```python
from build123d import *

# Parameters (mm, degrees)
SKETCH_1_R      = 2
EXTRUDE_1_DEPTH = 5.6
FILLET_1_R      = 2
FILLET_2_R      = 2
FILLET_3_R      = 50


with BuildPart() as part:
    # ｽｹｯﾁ1 → ﾎﾞｽ - 押し出し1 (new body)
    with BuildSketch(Plane(origin=(0, 0, 0), x_dir=(1, 0, 0), z_dir=(0, 1, 0))):
        with BuildLine():
            Line((47.5, -35), (67.5, -58.4))
            Line((67.5, -58.4), (67.5, -108.4))
            Line((67.5, -108.4), (36.64, -142.480487319))
            Line((36.64, -142.480487319), (36.64, -172))
            Line((36.64, -172), (-13.36, -172))
            Line((-13.36, -172), (-13.36, -106.551632211))
            ThreePointArc((-13.36, -106.551632211), (45.682817739, -101.546532593), (0, -63.808150114))
            Line((0, -63.808150114), (0, 0))
            Line((0, 0), (37.5, 0))
            Line((37.5, 0), (37.5, -15))
            Line((37.5, -15), (47.5, -15))
            Line((47.5, -15), (47.5, -35))
        make_face()
        with Locations(Location((42.5, -25, 0), (0, 0, 270))):
            Circle(SKETCH_1_R, mode=Mode.SUBTRACT)
        with Locations(Location((42.5, -51, 0), (0, 0, 270))):
            Circle(SKETCH_1_R, mode=Mode.SUBTRACT)
    extrude(amount=EXTRUDE_1_DEPTH)

    # ﾌｨﾚｯﾄ1
    fillet_1_edges = [part.edges().sort_by_distance(p)[0] for p in [
        (-13.36, 2.8, 106.551632211),
        (0, 2.8, 63.808150114),
    ]]
    fillet(fillet_1_edges, radius=FILLET_1_R)

    # ﾌｨﾚｯﾄ2
    fillet_2_edges = [part.edges().sort_by_distance(p)[0] for p in [
        (0, 2.8, 0),
        (37.5, 2.8, 0),
        (47.5, 2.8, 15),
        (67.5, 2.8, 58.4),
        (67.5, 2.8, 108.4),
        (36.64, 2.8, 172),
        (-13.36, 2.8, 172),
    ]]
    fillet(fillet_2_edges, radius=FILLET_2_R)

    # ﾌｨﾚｯﾄ3
    fillet_3_edges = [part.edges().sort_by_distance(p)[0] for p in [
        (36.64, 2.8, 142.480487319),
    ]]
    fillet(fillet_3_edges, radius=FILLET_3_R)


solid = part.part
```
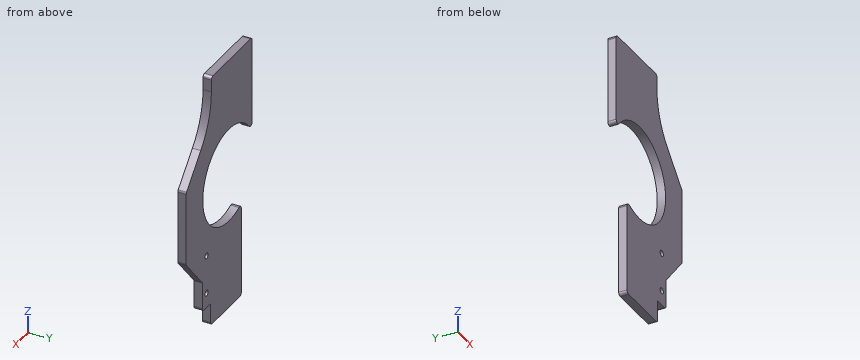
Read the model definition and answer for the solid it produces. Units are mm, in the model's axes. Coordinates: 2 decimals unless noted, no trailing zeros. Loops run counter-clockwise (first coordinate to the right, second up) from the corner with the lowest first, then second, coordinate; pieces in that order, holes last. Notation, with made-up numbers: (-12.75, 38) -> (36.25, 38) arc R35 ccw to (36.25, 75) -> close; hole circle Ø11 at (48, 31.5). An arc over 180 degrees is marked (long way). Return JSON: item names as keys, results as strings.
Item 1: Find section C-C (y = 1.55). Determine the outline of the cut face in (x, z).
Answers:
{"outline": "(-13.36, 113.3) arc R2 ccw to (-9.8, 112.05) arc R32 cw (long way) to (2.77, 62.49) arc R2 ccw to (0, 60.64) -> (0, 2) arc R2 ccw to (2, 0) -> (35.5, 0) arc R2 ccw to (37.5, 2) -> (37.5, 15) -> (45.5, 15) arc R2 ccw to (47.5, 17) -> (47.5, 35) -> (67.02, 57.84) arc R2 ccw to (67.5, 59.14) -> (67.5, 107.63) arc R2 ccw to (66.98, 108.97) -> (49.58, 128.19) arc R50 cw to (36.64, 161.75) -> (36.64, 170) arc R2 ccw to (34.64, 172) -> (-11.36, 172) arc R2 ccw to (-13.36, 170) -> close; hole circle Ø4 at (42.5, 25); hole circle Ø4 at (42.5, 51)"}
Item 2: Find section A-A (z = 25). Determine the outline of the cut face in (x, y), plus the area to 3 significant figures.
Answers:
{"outline": "(0, 0) -> (40.5, 0) -> (40.5, 5.6) -> (0, 5.6) -> close; (44.5, 0) -> (47.5, 0) -> (47.5, 5.6) -> (44.5, 5.6) -> close", "area": "244 mm2"}
Item 3: Find section D-D (x = 42.5). Determine the outline of the cut face in (y, z), plus the area to 3 significant figures.
Answers:
{"outline": "(0, 15) -> (5.6, 15) -> (5.6, 23) -> (0, 23) -> close; (0, 27) -> (5.6, 27) -> (5.6, 49) -> (0, 49) -> close; (0, 53) -> (5.6, 53) -> (5.6, 75.4) -> (0, 75.4) -> close; (0, 108.6) -> (5.6, 108.6) -> (5.6, 138.27) -> (0, 138.27) -> close", "area": "460 mm2"}
Item 4: Find the intervals of material crossed by probe 1 along X at (y, z) = (5.25, 25); probe 2 along X at (y, z) = (4.7, 121); probe 3 along Z at (x, y) = (18.5, 5.2), in increasing order.
Answers:
{"probe 1": "x = 0 to 40.5, 44.5 to 47.5", "probe 2": "x = -13.36 to 1.61, 28.67 to 56.09", "probe 3": "z = 0 to 60.18, 123.82 to 172"}
Item 5: Find section B-B (x = 4.5). Determine the outline of the cut face in (y, z), plus the area to 3 significant figures.
Answers:
{"outline": "(0, 0) -> (5.6, 0) -> (5.6, 61.82) -> (0, 61.82) -> close; (0, 122.18) -> (5.6, 122.18) -> (5.6, 172) -> (0, 172) -> close", "area": "625 mm2"}
Item 6: Flat-ended cylindrical pins translate along their axes: P1, Ø3, axis at x = 42.5, z = 25, coming from the +Y side; P2, Ø2, axis at y = 3, z = 19, coming from the +X side; P3, Ø5, axis at x = 29, z = 43, coming from the -Y side; P4, Ø2, axis at y = 1, z = 92.5, coming from the -X side. Find the tip coordinate at first contact, or state that the pin passes through.
Answers:
{"P1": "passes through", "P2": "stops at x = 47.5", "P3": "stops at y = 0", "P4": "stops at x = 47.1"}
